Work out the finished part from the listing and answer in its coordinate system (mm). Round coordinates to 2 decimals unless told otherwise and drop trailing zeros. Order: outer loops, then holes, each group sorted by start corner. A loop starts at its lowest first (then second) coordinate and runs counter-clockwise, first axis right, second up. Notation, with made-up numbers: M 50,24.25 L 61,24.25 A8 ccw 61,31.25 Z; hole C 16.25,82.25 d7. An arc over 180 degrees is marked long. Return JSON: item names as keys, results as strings.
Autodesk Inventor part; units mm, degrees
ref_plane "YZ Plane" through (0, 0, 0) normal (1, 0, 0) x (0, 1, 0)
ref_plane "XZ Plane" through (0, 0, 0) normal (0, 1, 0) x (-1, 0, 0)
ref_plane "XY Plane" through (0, 0, 0) normal (0, 0, 1) x (1, 0, 0)
sketch "Sketch1" plane through (0, 0, 0) normal (0, 1, 0) x (-1, 0, 0)
  line L0 (-22.05, -28.75) -> (22.05, -28.75)
  line L1 (22.05, -28.75) -> (22.05, 28.75)
  line L2 (22.05, 28.75) -> (-22.05, 28.75)
  line L3 (-22.05, 28.75) -> (-22.05, -28.75)
  line L4 (-22.05, -28.75) -> (22.05, 28.75) construction
  line L5 (22.05, -28.75) -> (-22.05, 28.75) construction
  point P0 (0, 0)
  dimension "d0" = 57.5
  dimension "d1" = 44.1
extrude "Extrusion1" add sketch "Sketch1" along normal blind 1.3
chamfer "Chamfer1" distance 2 angle 45 1 edges at (-22.05, 0.65, -28.75)
sketch "Sketch4" plane through (0, 1.3, 0) normal (0, 1, 0) x (1, 0, 0)
  line L0 (22.6381, -25.9185) -> (13.7388, -25.9185)
  line L1 (13.7388, -25.9185) -> (13.7388, -21.956)
  line L2 (13.7388, -21.956) -> (22.6381, -21.956)
  line L3 (22.6381, -21.956) -> (22.6381, -25.9185)
  line L4 (11.4165, -21.956) -> (0.7633, -21.956)
  line L5 (0.7633, -21.956) -> (0.7633, -24.4569)
  line L6 (0.7633, -24.4569) -> (11.4165, -24.4569)
  line L7 (11.4165, -24.4569) -> (11.4165, -21.956)
  line L8 (-0.6658, -26.6006) -> (-6.707, -26.6006)
  line L9 (-6.707, -26.6006) -> (-6.707, -22.3783)
  line L10 (-6.707, -22.3783) -> (-0.6658, -22.3783)
  line L11 (-0.6658, -22.3783) -> (-0.6658, -26.6006)
  line L12 (-6.707, -24.392) -> (-14.5426, -24.392)
  line L13 (-14.5426, -24.392) -> (-14.5426, -21.0953)
  line L14 (-14.5426, -21.0953) -> (-6.707, -21.0953)
  line L15 (-6.707, -21.0953) -> (-6.707, -24.392)
  line L16 (-14.5426, -21.0953) -> (-11.8996, -21.0953)
  line L17 (-11.8996, -21.0953) -> (-11.8996, -19.5363)
  line L18 (-11.8996, -19.5363) -> (-14.5426, -19.5363)
  line L19 (-14.5426, -19.5363) -> (-14.5426, -21.0953)
  line L20 (-21.1238, -24.2621) -> (-17.4211, -24.2621)
  line L21 (-17.4211, -24.2621) -> (-17.4211, -21.956)
  line L22 (-17.4211, -21.956) -> (-21.1238, -21.956)
  line L23 (-21.1238, -21.956) -> (-21.1238, -24.2621)
  line L24 (5.6616, -20.7705) -> (1.894, -20.7705)
  line L25 (1.894, -20.7705) -> (1.894, -17.3277)
  line L26 (1.894, -17.3277) -> (5.6616, -17.3277)
  line L27 (5.6616, -17.3277) -> (5.6616, -20.7705)
  line L28 (-2.848, -19.9261) -> (-5.2515, -19.9261)
  line L29 (-5.2515, -19.9261) -> (-5.2515, -18.3346)
  line L30 (-5.2515, -18.3346) -> (-2.848, -18.3346)
  line L31 (-2.848, -18.3346) -> (-2.848, -19.9261)
  line L32 (-17.2689, -17.0029) -> (-14.5426, -17.0029)
  line L33 (-14.5426, -17.0029) -> (-14.5426, -13.4952)
  line L34 (-14.5426, -13.4952) -> (-17.2689, -13.4952)
  line L35 (-17.2689, -13.4952) -> (-17.2689, -17.0029)
  line L36 (15.925, -11.4814) -> (12.4173, -11.4814)
  line L37 (12.4173, -11.4814) -> (12.4173, -14.7294)
  line L38 (12.4173, -14.7294) -> (15.925, -14.7294)
  line L39 (15.925, -14.7294) -> (15.925, -11.4814)
  line L40 (-2.1335, 9.0455) -> (1.894, 9.0455)
  line L41 (1.894, 9.0455) -> (1.894, -8.9481)
  line L42 (1.894, -8.9481) -> (-2.1335, -8.9481)
  line L43 (-2.1335, -8.9481) -> (-2.1335, 9.0455)
  line L44 (4.5573, 3.3291) -> (1.6991, 3.3291)
  line L45 (1.6991, 3.3291) -> (1.6991, 0.6009)
  line L46 (1.6991, 0.6009) -> (4.5573, 0.6009)
  line L47 (4.5573, 0.6009) -> (4.5573, 3.3291)
  line L48 (-17.5287, 13.7631) -> (-14.1519, 13.7631)
  line L49 (-14.1519, 13.7631) -> (-14.1519, 10.4096)
  line L50 (-14.1519, 10.4096) -> (-17.5287, 10.4096)
  line L51 (-17.5287, 10.4096) -> (-17.5287, 13.7631)
  line L52 (16.8052, 16.3739) -> (14.7212, 16.3739)
  line L53 (14.7212, 16.3739) -> (14.7212, 12.4259)
  line L54 (14.7212, 12.4259) -> (16.8052, 12.4259)
  line L55 (16.8052, 12.4259) -> (16.8052, 16.3739)
  line L56 (-23.3919, 26.0219) -> (-13.2211, 26.0219)
  line L57 (-13.2211, 26.0219) -> (-13.2211, 21.0711)
  line L58 (-13.2211, 21.0711) -> (-23.3919, 21.0711)
  line L59 (-23.3919, 21.0711) -> (-23.3919, 26.0219)
  line L60 (-20.3793, 16.7032) -> (-17.8455, 16.7032)
  line L61 (-17.8455, 16.7032) -> (-17.8455, 19.4346)
  line L62 (-17.8455, 19.4346) -> (-20.3793, 19.4346)
  line L63 (-20.3793, 19.4346) -> (-20.3793, 16.7032)
  line L64 (-11.5832, 21.8169) -> (-0.7032, 21.8169)
  line L65 (-0.7032, 21.8169) -> (-0.7032, 24.5446)
  line L66 (-0.7032, 24.5446) -> (-11.5832, 24.5446)
  line L67 (-11.5832, 24.5446) -> (-11.5832, 21.8169)
  line L68 (-2.5673, 18.6812) -> (-4.8458, 18.6812)
  line L69 (-4.8458, 18.6812) -> (-4.8458, 22.2038)
  line L70 (-4.8458, 22.2038) -> (-2.5673, 22.2038)
  line L71 (-2.5673, 22.2038) -> (-2.5673, 18.6812)
  line L72 (0.9146, 27.1153) -> (6.539, 27.1153)
  line L73 (6.539, 27.1153) -> (6.539, 22.2038)
  line L74 (6.539, 22.2038) -> (0.9146, 22.2038)
  line L75 (0.9146, 22.2038) -> (0.9146, 27.1153)
  line L76 (2.2307, 17.9158) -> (4.5573, 17.9158)
  line L77 (4.5573, 17.9158) -> (4.5573, 22.2038)
  line L78 (4.5573, 22.2038) -> (2.2307, 22.2038)
  line L79 (2.2307, 22.2038) -> (2.2307, 17.9158)
  line L80 (6.0899, 24.1958) -> (14.5454, 24.1958)
  line L81 (14.5454, 24.1958) -> (14.5454, 21.5323)
  line L82 (14.5454, 21.5323) -> (6.0899, 21.5323)
  line L83 (6.0899, 21.5323) -> (6.0899, 24.1958)
  line L84 (14.2886, 21.5323) -> (11.9019, 21.5323)
  line L85 (11.9019, 21.5323) -> (11.9019, 19.3557)
  line L86 (11.9019, 19.3557) -> (14.2886, 19.3557)
  line L87 (14.2886, 19.3557) -> (14.2886, 21.5323)
  line L88 (21.4363, 24.0758) -> (17.64, 24.0758)
  line L89 (17.64, 24.0758) -> (17.64, 21.5323)
  line L90 (17.64, 21.5323) -> (21.4363, 21.5323)
  line L91 (21.4363, 21.5323) -> (21.4363, 24.0758)
  line L92 (12.1107, -20.099) -> (10.5174, -18.49)
  line L93 (10.5174, -18.49) -> (11.3144, -17.7008)
  line L94 (11.3144, -17.7008) -> (12.9077, -19.3099)
  line L95 (12.9077, -19.3099) -> (12.1107, -20.099)
  line L96 (-18.9518, -11.1888) -> (-13.5356, -11.1888)
  line L97 (-13.5356, -11.1888) -> (-13.5356, -8.0664)
  line L98 (-13.5356, -8.0664) -> (-18.9518, -8.0664)
  line L99 (-18.9518, -8.0664) -> (-18.9518, -11.1888)
  point P0 (0, 0)
  point P1 (6.539, 24.1958)
  point P2 (6.0899, 22.2038)
extrude "Clearance Cutouts" cut sketch "Sketch4" against normal blind 1.5
sketch "Sketch5" plane through (0, 1.3, 0) normal (0, 1, 0) x (1, 0, 0)
  line L0 (9.9457, 22.5156) -> (-6.9835, 22.5156) construction
  line L1 (9.9457, 17.9158) -> (-6.9835, 17.9158)
  line L2 (-6.9835, 27.1153) -> (9.9457, 27.1153)
  arc A0 (9.9457, 17.9158) -> (9.9457, 27.1153) centre (9.9457, 22.5156) ccw
  arc A1 (-6.9835, 27.1153) -> (-6.9835, 17.9158) centre (-6.9835, 22.5156) ccw
  line L3 (-11.5832, 24.5446) -> (-0.7032, 24.5446)
  line L4 (0.9146, 22.2038) -> (0.9146, 27.1153)
  line L5 (-13.2211, 26.0219) -> (-13.2211, 21.0711)
  line L6 (-11.5832, 21.8169) -> (-11.5832, 24.5446)
  line L7 (14.5454, 24.1958) -> (14.5454, 21.5323)
  line L8 (-10.0926, -22.1506) -> (6.9665, -22.1506) construction
  line L9 (-10.0926, -26.6006) -> (6.9665, -26.6006)
  line L10 (6.9665, -17.7006) -> (-10.0926, -17.7006)
  arc A2 (-10.0926, -17.7006) -> (-10.0926, -26.6006) centre (-10.0926, -22.1506) ccw
  arc A3 (6.9665, -26.6006) -> (6.9665, -17.7006) centre (6.9665, -22.1506) ccw
  point P0 (0, 0)
  point P1 (1.4811, 22.5156)
  point P2 (14.5454, 22.5156)
  point P3 (-11.5832, 22.5156)
  point P4 (4.5573, 17.9158)
  point P5 (-1.5631, -22.1506)
  point P6 (-0.6658, -26.6006)
  point P7 (11.4165, -22.1506)
  point P8 (11.4165, -24.4569)
  point P9 (-14.5426, -22.1506)
  point P10 (-14.5426, -19.5363)
  dimension "d53" = 8.9
extrude "Extrusion4" cut sketch "Sketch5" against normal blind 1.5 contours L1 A1 L2 A0 | A2 L10 A3 L9
sketch "Sketch6" plane through (0, 0, 0) normal (0, -1, 0) x (1, 0, 0)
  line L0 (22.05, 21.956) -> (22.05, -28.75)
  line L1 (22.05, -16.5) -> (-12.45, -16.5)
  line L2 (-12.45, -16.5) -> (-12.45, 16.5)
  line L3 (-12.45, 16.5) -> (22.05, 16.5)
  line L4 (22.05, 16.5) -> (22.05, -16.5)
  point P0 (0, 0)
  point P1 (22.05, 16.5)
  dimension "d44" = 33
  dimension "d45" = 34.5
  dimension "d46" = 16.5
extrude "Extrusion5" cut sketch "Sketch6" against normal through all
sketch "Sketch7" plane through (0, 1.3, 0) normal (0, 1, 0) x (1, 0, 0)
  line L0 (-22.05, -28.75) -> (22.05, -28.75)
  arc A0 (4, -28.75) -> (-4, -28.75) centre (0, -28.75) ccw
  line L1 (22.05, 28.75) -> (-20.05, 28.75)
  arc A1 (-4, 28.75) -> (4, 28.75) centre (0, 28.75) ccw
  line L2 (22.05, 28.75) -> (-20.05, 28.75)
  point P0 (0, 0)
  point P1 (4, 28.75)
  dimension "d49" = 4
  dimension "d50" = 4
extrude "Extrusion6" add sketch "Sketch7" against normal up to surface (1.3 mm away)
equation "\"d50\" = d49"
properties part number "Flex Holder V1" material "Thermoplastic Resin"
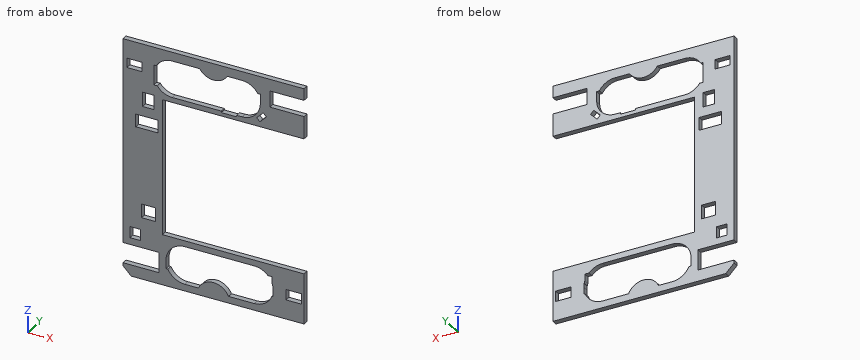
Item 1: Find section A-A (x = 15.5). Determine the outline of the cut face in (y, z), plus the area to 3 significant figures.
Output:
{"outline": "M 0,-28.75 L 1.3,-28.75 L 1.3,-16.5 L 0,-16.5 Z; M 0,16.5 L 1.3,16.5 L 1.3,21.96 L 0,21.96 Z; M 0,25.92 L 1.3,25.92 L 1.3,28.75 L 0,28.75 Z", "area": "26.7 mm^2"}
Item 2: Each of these flat-tipped pins is pushed along its axis until it touches: pin 1 (10 mm diameter, centred on x = -5, z = 10, fed in from -Y); pin 2 (0.6 mm diameter, centred on y = 0.5, z = 15.5, fed in from +X). Where does it stop, or does it pass through?
Output:
{"pin 1": "passes through", "pin 2": "stops at x = -12.45"}
Item 3: Find section D-D (y = 0.85). State how many separate pieces and enclosed holes the cut face has, plus the area to 3 significant figures.
Output:
{"separate pieces": "1", "enclosed holes": "9", "area": "834 mm^2"}
Item 4: Find section C-C (x = 8). Determine the outline of the cut face in (y, z).
Output:
{"outline": "M 0,-28.75 L 1.3,-28.75 L 1.3,-27.12 L 0,-27.12 Z; M 0,-17.92 L 1.3,-17.92 L 1.3,-16.5 L 0,-16.5 Z; M 0,16.5 L 1.3,16.5 L 1.3,17.82 L 0,17.82 Z; M 0,26.48 L 1.3,26.48 L 1.3,28.75 L 0,28.75 Z"}
Item 5: Consider line 1 along Z through (x, y) = (-5, 0.2); line 2 along Z through (x, y) = (-19, 1.25); line 3 along Z through (x, y) = (-18, 0.75). Determine where each line is inside the solid, lowest interval first. Write a range as [from, to].
Output:
{"line 1": "z = [-28.75, -27.12], [-17.92, -16.5], [16.5, 17.7], [26.6, 28.75]", "line 2": "z = [-28.75, -26.02], [-21.07, -19.43], [-16.7, 21.96], [24.26, 28.75]", "line 3": "z = [-28.75, -26.02], [-21.07, -19.43], [-16.7, 8.07], [11.19, 21.96], [24.26, 28.75]"}
Item 6: Find section B-B (z = 9.5). Determine the outline of the cut face in (x, y).
Output:
{"outline": "M -22.05,0 L -18.95,0 L -18.95,1.3 L -22.05,1.3 Z; M -13.54,0 L -12.45,0 L -12.45,1.3 L -13.54,1.3 Z"}
